Design review of the part built by this model. Coordinates are the model's own, in mm. A direction names the side the tool comes from. Round coordinates to 2 decimals unless told otherwise and drop trailing zeros. Loops run counter-clockwise (first coordinate to the right, second up) from the corner with the lowest first, then second, coordinate; pieces in that order, holes last. Notation, with made-up numbers: M -38.5,60 L -28.5,60 A20 ccw -28.5,73 Z; hole C 62,29 d5. An arc over 180 degrees is marked long. Answer as CSV lines item,"result". Start each with the question number.
from build123d import *

# Parameters (mm, degrees)
BOSS_EXTRUDE1_DEPTH = 5.875
CHAMFER1_SIZE       = 1
SKETCH2_R           = 2.1
CUT_EXTRUDE1_DEPTH  = 22.5
SKETCH3_R           = 4.25
CUT_EXTRUDE2_DEPTH  = 6.5


with BuildPart() as part:
    # Sketch1 → Boss-Extrude1 (new body, symmetric)
    with BuildSketch(Plane(origin=(0, 0, 0), x_dir=(1, 0, 0), z_dir=(0, 1, 0))):
        with BuildLine():
            Line((-21.5, 0), (-13.29, 0))
            ThreePointArc((-13.29, 0), (0, 13.29), (13.29, 0))
            Line((13.29, 0), (21.5, 0))
            ThreePointArc((21.5, 0), (0, 21.5), (-21.5, 0))
        make_face()
    extrude(amount=BOSS_EXTRUDE1_DEPTH, both=True)

    # Chamfer1
    chamfer1_edges = [part.edges().sort_by_distance(p)[0] for p in [
        (0, 5.875, -21.5),
    ]]
    chamfer(chamfer1_edges, length=CHAMFER1_SIZE)

    # Sketch2 → Cut-Extrude1 (cut, through all)
    with BuildSketch(Plane.XY):
        with Locations((-17.25, -1.125)):
            Circle(SKETCH2_R)
        with Locations((17.25, -1.125)):
            Circle(SKETCH2_R)
    extrude(amount=-CUT_EXTRUDE1_DEPTH, mode=Mode.SUBTRACT)

    # Sketch3 → Cut-Extrude2 (cut)
    with BuildSketch(Plane.XY):
        with Locations((-9, -0.5)):
            Circle(SKETCH3_R)
        with Locations((9, -0.5)):
            Circle(SKETCH3_R)
    extrude(amount=-CUT_EXTRUDE2_DEPTH, mode=Mode.SUBTRACT)


solid = part.part
Item 1: Consider section A-A, the plane y = -2.5. Write out the cut boundary in (x, z), then the cut area to 3 significant figures.
Item 2: To check wall thickness, follow line 1 (Y direction, x = 17.25, z = -7.25) (3 decimals); line 2 (X direction, y = -2.75, z = -1.5); line 3 (X direction, y = -2.75, z = -4). State the ranges of each line that lie inside material, in increasing order.
Item 3: Consider section C-C, the plane x = 0. Write out the cut boundary in (y, z) (3 decimals).
Item 4: Tool access review of faces 4 (the face through (-0.292, 0.082, -13.287)), 5 (the face through (13.25, -0.55, -4.33)): name each direction out of +Z, -Z, +X, -X, +Y, -Y from which nothing blocks a thin tool from reaching the whole face with its end or side.
Item 5: Consider section D-D, the plane y = -4.5. Write out the cut boundary in (x, z).
Item 6: Consider section B-B, the plane z = -7.75. Count the separate pieces of the cut face and the enclosed holes in it, then the cut area to 3 significant figures.
Item 7: The part is to be moulded in two halves that separate along X. For faces 1 (the face through (0.45, 5.72, -20.65)), 2 (the face through (0, -5.875, -16)), 3 (the face through (12, 0, -6.5)), say which applies: +X half, -X half, draft (parallel to the pull), parting line (faces both ways), or undercut.
Item 8: Insertion check: pin 1 Ø0.8 at (x, y) = (12.5, 0) entering from +Z; pin 2 Ø12 at (x, z) = (-3.5, -3) entering from +Y. Each pin has a flat end and moves straight along its axis. Give the tip position at first contact, or say it passes through.
Found:
1,outline,"M -21.5,0 A21.5 ccw -18.84,-10.36 L -18.84,0 Z; M -15.66,-14.73 A21.5 ccw 15.66,-14.73 L 15.66,0 L 13.29,0 A13.29 cw 12.75,-3.75 L 12.75,-6.5 L 11.59,-6.5 A13.29 cw -11.59,-6.5 L -12.75,-6.5 L -12.75,-3.75 A13.29 cw -13.29,0 L -15.66,0 Z; M 18.84,-10.36 A21.5 ccw 21.5,0 L 18.84,0 Z"
1,area,"365 mm^2"
2,line 1,"y = -5.875 to -3.225, 0.975 to 5.875"
2,line 2,"x = -21.45 to -18.58, -15.92 to -13.21, 13.21 to 15.92, 18.58 to 21.45"
2,line 3,"x = -21.12 to -18.58, -15.92 to -12.67, 12.67 to 15.92, 18.58 to 21.12"
3,outline,"M -5.875,-21.5 L 4.875,-21.5 L 5.875,-20.5 L 5.875,-13.29 L -5.875,-13.29 Z"
4,face 4,"+Z, +Y, -Y"
4,face 5,"+Z"
5,outline,"M -21.5,0 A21.5 ccw 21.5,0 L 13.29,0 A13.29 cw -13.29,0 Z"
6,separate pieces,"2"
6,enclosed holes,"2"
6,area,"189 mm^2"
7,face 1,"parting line"
7,face 2,"draft"
7,face 3,"undercut"
8,pin 1,"stops at z = -6.5"
8,pin 2,"passes through"
